from build123d import *

# Parameters (mm, degrees)
SKETCH1_R                       = 5
EXTRUDE_L3_DEPTH                = 30
CLAW_EXTRUDE_DEPTH              = 10
THREAD_TO_CLAW_JOINING_FILLET_R = 0.8
SKETCH9_R                       = 5
CLEVIS_HOLE_DEPTH               = 1.0000001
CLEVIS_HOLE_DEPTH_BACK          = 21.0000001
CLEVIS_HOLE_CHAMFER_SIZE        = 0.5


with BuildPart() as part:
    # Sketch1 → L3 (new body)
    with BuildSketch(Plane(origin=(0, 0, 0), x_dir=(0, 0, -1), z_dir=(1, 0, 0))):
        Circle(SKETCH1_R)
    extrude(amount=EXTRUDE_L3_DEPTH)

    # Sketch6 → Claw Extrude (add, symmetric)
    with BuildSketch(Plane.XY):
        Polygon((30, -10), (30, 10), (69, 10), (69, 5), (37, 5), (37, -5), (69, -5), (69, -10), align=None)
    extrude(amount=CLAW_EXTRUDE_DEPTH, both=True)

    # Sketch8 → Claw Bevelling (revolve, cut)
    with BuildSketch(Plane(origin=(0, 0, 0), x_dir=(1, 0, 0), z_dir=(0, 1, 0))):
        Polygon((30, 5), (55.980762114, 50), (30, 50), align=None)
    revolve(axis=Axis((-49.725315437, 0, 0), (1, 0, 0)), mode=Mode.SUBTRACT)

    # Thread to Claw Joining Fillet
    thread_to_claw_joining_fillet_edges = [part.edges().sort_by_distance(p)[0] for p in [
        (30, 0, 5),
    ]]
    fillet(thread_to_claw_joining_fillet_edges, radius=THREAD_TO_CLAW_JOINING_FILLET_R)

    # Sketch11 → Claw Conic Taper (revolve, cut)
    with BuildSketch(Plane.XY):
        Polygon((11.264973081, 105), (69, 5), (69, 105), align=None)
    revolve(axis=Axis((56.222491899, 0, 0), (-1, 0, 0)), mode=Mode.SUBTRACT)

    # Sketch9 → Clevis Hole (cut, two sides)
    with BuildSketch(Plane(origin=(0, 10, 0), x_dir=(1, 0, 0), z_dir=(0, 1, 0))) as clevis_hole_sk:
        with Locations((57, 0)):
            Circle(SKETCH9_R)
    extrude(amount=CLEVIS_HOLE_DEPTH, mode=Mode.SUBTRACT)
    extrude(clevis_hole_sk.sketch, amount=-CLEVIS_HOLE_DEPTH_BACK, mode=Mode.SUBTRACT)

    # Clevis Hole Chamfer
    clevis_hole_chamfer_edges = [part.edges().sort_by_distance(p)[0] for p in [
        (52, -10, 0),
        (52, 10, 0),
    ]]
    chamfer(clevis_hole_chamfer_edges, length=CLEVIS_HOLE_CHAMFER_SIZE)

    # Sketch23 → Thread End Chamf (revolve, cut)
    with BuildSketch(Plane.XY):
        Polygon((0, 4.08), (0, 5), (0.531162248, 5), align=None)
    revolve(axis=Axis((-11.219306213, 0, 0), (1, 0, 0)), mode=Mode.SUBTRACT)


solid = part.part
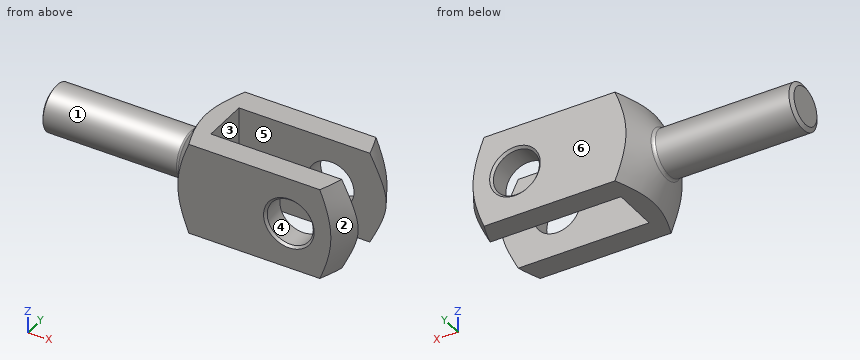
The model under review builds one solid part; all positions refer to its coordinate system, in mm. Face numbers are marked on the shaded views. A direction names the side the tool comes from. Round coordinates to 2 decimals unless told otherwise and drop trailing zeros. Write each loop counter-clockwise with the first axis right and the second up, starting at its lowest first coordinate (ties: lowest second). Pieces come first, ordered by that corner, then holes. Notation, with made-up numbers: (-2.75, 22.5) -> (3.25, 22.5) arc R10 ccw to (3.25, 36.5) -> close; hole circle Ø8 at (-3, -39). An arc over 180 degrees is marked (long way). Answer as a JSON object with one key per item and string values.
1. Machinability: for the marked faces 5 and 6, which of the approach directions +Z, -Z, +X, -X, +Y, -Y give a long, thin tool a straight path to every point of the face, cutting with its end or side? Answer none if there is none.
Results found:
{"face 5": "+Z, -Z, +X", "face 6": "+Z, -Z, +X, -X, +Y"}
2. To check wall thickness, follow line 1 along Y through (x, z) = (43.5, 2); line 2 along X through (y, z) = (2.75, 2). State the ranges of each line that lie inside material, in increasing order.
Results found:
{"line 1": "y = -10 to -5, 5 to 10", "line 2": "x = 0 to 37"}
3. We need section D-D on x = 7.5. State the section outline as (y, z) points.
Results found:
{"outline": "circle Ø10 at (0, 0)"}
4. The part is to be moulded in two halves that separate along Y. For the marked faces 1, 2, 3 and 4, say which applies: pulls with the +Y half, pulls with the -Y half, needs draft (parallel to the pull), parting line crosses it, or undercut.
Results found:
{"face 1": "parting line crosses it", "face 2": "pulls with the -Y half", "face 3": "undercut", "face 4": "needs draft"}
5. Clearance check with flat-ended pins moving along their axes: pin 1 (1.5 mm diameter, centred on x = 7.5, y = -6, fed in from +Z) (3 decimals); pin 2 (1 mm diameter, centred on y = 5, z = 6, fed in from -X); pin 3 (1 mm diameter, centred on x = 18, y = 0, fed in from +Z); pin 4 (10 mm diameter, centred on x = 27.5, z = -6.5, fed in from +Y). State where each tip first meets the part, or that it passes through.
Results found:
{"pin 1": "passes through", "pin 2": "stops at x = 31.33", "pin 3": "stops at z = 5", "pin 4": "stops at y = 7.4"}
6. We need section A-A on x = 44. State the section outline as (y, z) points, and give its area (3 significant figures).
Results found:
{"outline": "(-10, -10) -> (-5, -10) -> (-5, 10) -> (-10, 10) -> close; (5, -10) -> (10, -10) -> (10, 10) -> (5, 10) -> close", "area": "200 mm^2"}
7. We need section B-B on x = 57. State the section outline as (y, z) points, and give its area (3 significant figures).
Results found:
{"outline": "(-10, -10) -> (-5, -10) -> (-5, -5) -> (-9.5, -5) -> (-10, -5.5) -> close; (-10, 5.5) -> (-9.5, 5) -> (-5, 5) -> (-5, 10) -> (-10, 10) -> close; (5, -10) -> (10, -10) -> (10, -5.5) -> (9.5, -5) -> (5, -5) -> close; (5, 5) -> (9.5, 5) -> (10, 5.5) -> (10, 10) -> (5, 10) -> close", "area": "99.5 mm^2"}
8. We need section C-C on z = 0. State how many separate pieces and enclosed holes the cut face has, and give its area (3 significant figures).
Results found:
{"separate pieces": "3", "enclosed holes": "0", "area": "630 mm^2"}
